from build123d import *

# Parameters (mm, degrees)
BOSS_EXTRUDE1_DEPTH     = 38.1
SKETCH3_W               = 15.113
SKETCH3_H               = 6.477
CUT_EXTRUDE3_DEPTH      = 100.886424174
SKETCH4_W               = 22.86
SKETCH4_H               = 3.81
CUT_EXTRUDE4_DEPTH      = 108.200359108
SKETCH5_R               = 10.8585
CUT_EXTRUDE5_DEPTH      = 25.4
FILLET1_R               = 6.35
CUT_EXTRUDE6_DEPTH      = 110.286380048
CUT_EXTRUDE6_DEPTH_BACK = 110.286380048
SKETCH6_R               = 1.349999967
FILLET2_R               = 5.08


with BuildPart() as part:
    # Sketch1 → Boss-Extrude1 (new body)
    with BuildSketch(Plane(origin=(0, 0, 0), x_dir=(1, 0, 0), z_dir=(0, 1, 0))):
        Polygon((0, 0), (-31.5214, 0), (-31.5214, 30.226), (-58.462168363, 57.166768363), (-31.5214, 84.107536726), (6.5786, 46.007536726), (6.5786, 21.59), (0, 21.59), align=None)
    extrude(amount=BOSS_EXTRUDE1_DEPTH)

    # Sketch3 → Cut-Extrude3 (cut, through all)
    with BuildSketch(Plane.ZY.offset(31.5214)):
        Polygon((-15.113, 27.813), (-15.113, 31.623), (-15.113, 38.1), (-21.59, 38.1), (-21.59, 27.813), align=None)
        with Locations((-7.5565, 34.8615)):
            Rectangle(SKETCH3_W, SKETCH3_H)
        Polygon((-21.59, 10.287), (-21.59, 0), (-15.113, 0), (-15.113, 6.477), (-15.113, 10.287), align=None)
        with Locations((-7.5565, 3.2385)):
            Rectangle(SKETCH3_W, SKETCH3_H)
    extrude(amount=-CUT_EXTRUDE3_DEPTH, mode=Mode.SUBTRACT)

    # Sketch4 → Cut-Extrude4 (cut, through all)
    with BuildSketch(Plane.XZ.offset(-6.477)):
        with Locations((-14.732, -11.95324)):
            Rectangle(SKETCH4_W, SKETCH4_H)
    extrude(amount=-CUT_EXTRUDE4_DEPTH, mode=Mode.SUBTRACT)

    # Sketch5 → Cut-Extrude5 (cut)
    with BuildSketch(Plane(origin=(-57.814468363, 0, -57.814468363), x_dir=(-0.7071067811865489, 0, 0.7071067811865462), z_dir=(-0.7071067811865462, 0, -0.7071067811865489))):
        with Locations((-18.134013876, 19.05)):
            Circle(SKETCH5_R)
    extrude(amount=-CUT_EXTRUDE5_DEPTH, mode=Mode.SUBTRACT)

    # Fillet1
    fillet1_edges = [part.edges().sort_by_distance(p)[0] for p in [
        (-31.5214, 19.05, -30.226),
        (6.5786, 19.05, -46.007536726),
    ]]
    fillet(fillet1_edges, radius=FILLET1_R)

    # Sketch6 → Cut-Extrude6 (cut, two sides: drawn at the far end of the back side and taken through both)
    with BuildSketch(Plane(origin=(0, 38.1, 0), x_dir=(1, 0, 0), z_dir=(0, 1, 0)).offset(-CUT_EXTRUDE6_DEPTH_BACK)):
        with Locations(Location((-36.011528061, 61.656896424, 0), (0, 0, 270))):
            Circle(SKETCH6_R)
    extrude(amount=CUT_EXTRUDE6_DEPTH + CUT_EXTRUDE6_DEPTH_BACK, mode=Mode.SUBTRACT)

    # Fillet2
    fillet2_edges = [part.edges().sort_by_distance(p)[0] for p in [
        (-58.462168363, 19.05, -57.166768363),
        (-31.5214, 19.05, -84.107536726),
        (-44.991784182, 38.1, -70.637152545),
        (-44.991784182, 0, -70.637152545),
    ]]
    fillet(fillet2_edges, radius=FILLET2_R)


solid = part.part
The listing builds one solid part. Answer for the finished solid, in the listing's coordinates (mm). A direction names the side the tool comes from. Coordinates: 2 decimals unless noted, no trailing zeros. Loops run counter-clockwise (first coordinate to the right, second up) from the corner with the lowest first, then second, coordinate; pieces in that order, holes last. Notation, with made-up numbers: M 87,19.25 L 106,19.25 A18 ccw 106,31.25 Z; hole C -13.5,68.5 d1. An arc over 180 degrees is marked long. Answer in a Markdown table with one row per item.
1) Determine the mould class of faces 4 (the flat face through (-24, 0, -45)), 5 (the cylindrical face through (-56.358, 19.317, -57.223)), 6 (the flat face through (-16, 8, -15.113)), 7 (the flat face through (-11.834, 18.783, -64.42)) for opening direction Z: released by +Z, released by -Z, zero draft, split by the parting line, or undercut.
Answers below:
| item | result |
|---|---|
| face 4 | zero draft |
| face 5 | split by the parting line |
| face 6 | undercut |
| face 7 | released by -Z |
2) Find section D-D (y = 35). Determine the outline of the cut face in (x, z), then the cut area to 3 significant figures.
Answers below:
| item | result |
|---|---|
| outline | M -55.99,-59.07 L -33.43,-81.63 A5.08 ccw -27.93,-80.52 L 4.72,-47.87 A6.35 ccw 6.58,-43.38 L 6.58,-21.59 L -31.52,-21.59 L -31.52,-27.6 A6.35 cw -33.38,-32.09 L -54.87,-53.57 A5.08 ccw Z; hole C -36.01,-61.66 d2.7 |
| area | 2,350 mm^2 |
3) Given pin 1 (1.1 mm diameter, centred on x = -19.5, y = 7.5, fed in from -Z); pin 2 (17.5 mm diameter, centred on y = 21, z = -10, fed in from +X); pin 3 (1.9 mm diameter, centred on x = -21, y = 29.5, fed in from -Z); pin 4 (1.6 mm diameter, centred on x = -36.01, z = -61.66, fed in from -Y), each flat-ended and moving along its own axis, determine where each tip first touches the part or whether it passes through.
Answers below:
| item | result |
|---|---|
| pin 1 | z = -72.64 |
| pin 2 | x = 0 |
| pin 3 | z = -74.54 |
| pin 4 | through |
4) Find section A-A (y = 24). Determine the outline of the cut face in (x, z).
Answers below:
| item | result |
|---|---|
| outline | M -54.87,-60.76 L -51.83,-63.8 L -33.87,-45.84 L -20.2,-59.51 L -38.16,-77.47 L -35.11,-80.52 A5.08 ccw -27.93,-80.52 L 4.72,-47.87 A6.35 ccw 6.58,-43.38 L 6.58,-21.59 L 0,-21.59 L 0,0 L -31.52,0 L -31.52,-27.6 A6.35 cw -33.38,-32.09 L -54.87,-53.57 A5.08 ccw Z; hole M -26.16,-13.86 L -3.3,-13.86 L -3.3,-10.05 L -26.16,-10.05 Z |
5) Find the intervals of material crossed by probe 1 along Z at (x, y) = (-24.5, 17); probe 2 along Z at (x, y) = (-10.5, 12); probe 3 along Z at (x, y) = (-37, 32), in increasing order.
Answers below:
| item | result |
|---|---|
| probe 1 | -77.09 to -65.23, -55.21 to -13.86, -10.05 to 0 |
| probe 2 | -63.09 to -13.86, -10.05 to 0 |
| probe 3 | -78.63 to -62.58, -60.74 to -35.7 |
6) Find section C-C (z = -23). Determine the outline of the cut face in (x, y), then the cut area to 3 significant figures.
Answers below:
| item | result |
|---|---|
| outline | M -31.52,0 L 6.58,0 L 6.58,38.1 L -31.52,38.1 Z |
| area | 1,450 mm^2 |
7) Find section B-B (x = -23). Count the separate pieces of the cut face and the enclosed holes in it, then the cut area to 3 significant figures.
Answers below:
| item | result |
|---|---|
| separate pieces | 2 |
| enclosed holes | 1 |
| area | 2,360 mm^2 |
8) Which of the six approach directions +Z, -Z, +X, -X, +Y, -Y give full straight-line access (tool end or side, diameter ignored) to faces 1 (the flat face through (-13, 32, -21.59)), 2 (the flat face through (-26.924, 19.202, -52.784)), 3 (the flat face through (-3.302, 19, -12))?
Answers below:
| item | result |
|---|---|
| face 1 | +X |
| face 2 | none |
| face 3 | +Y, -Y |
